Geometry check sheet. Reference: the model listing, model coordinates, mm. A direction names the side the tool comes from. Coordinates: 2 decimals unless noted, no trailing zeros. Write each loop counter-clockwise with the first axis right and the second up, starting at its lowest first coordinate (ties: lowest second). Pieces come first, ordered by that corner, then holes. Notation, with made-up numbers: M 76,-19 L 103,-19 A24 ccw 103,2 Z; hole C -36.5,61 d8. An arc over 180 degrees is marked long. Write each question's results on one line, items separated by ' | '.
```python
from build123d import *


with BuildPart() as part:
    # Sketch1 → Revolve1 (revolve)
    with BuildSketch(Plane.XY):
        with BuildLine():
            Line((1, 16.75), (0, 15.75))
            Line((0, 15.75), (0, 5.1))
            Line((0, 5.1), (15, 5.1))
            Line((15, 5.1), (15, 13.249667434))
            ThreePointArc((15, 13.249667434), (15.22452816, 13.805394131), (15.772080403, 14.049180096))
            Line((15.772080403, 14.049180096), (43, 15))
            Line((43, 15), (43, 19.5))
            ThreePointArc((43, 19.5), (42.121320344, 21.621320344), (40, 22.5))
            Line((40, 22.5), (9.28444402, 22.5))
            Line((9.28444402, 22.5), (5, 19.5))
            Line((5, 19.5), (5, 17.75))
            Line((5, 17.75), (3, 17.75))
            Line((3, 17.75), (3, 16.75))
            Line((3, 16.75), (1, 16.75))
        make_face()
    revolve(axis=Axis((0, 0, 0), (1, 0, 0)))


solid = part.part
```
Q1. Sectioned sample at A-A on y = 0. Record the cut outline in (x, z).
Geometry check:
outline: M 0,-15.75 L 1,-16.75 L 3,-16.75 L 3,-17.75 L 5,-17.75 L 5,-19.5 L 9.28,-22.5 L 40,-22.5 A3 ccw 43,-19.5 L 43,-15 L 15.77,-14.05 A0.8 cw 15,-13.25 L 15,-5.1 L 0,-5.1 Z; M 0,5.1 L 15,5.1 L 15,13.25 A0.8 cw 15.77,14.05 L 43,15 L 43,19.5 A3 ccw 40,22.5 L 9.28,22.5 L 5,19.5 L 5,17.75 L 3,17.75 L 3,16.75 L 1,16.75 L 0,15.75 Z
Q2. Scan lines: probe 1 along Z at (x, y) = (10, 0); probe 2 along Z at (x, y) = (7, 0); probe 3 along X at (y, z) = (-2.5, -5.5). Record each from-to range of solid material in increasing order.
Geometry check:
probe 1: z = -22.5 to -5.1, 5.1 to 22.5 | probe 2: z = -20.9 to -5.1, 5.1 to 20.9 | probe 3: x = 0 to 15
Q3. Sectioned sample at D-D on x = 25. Record the cut outline in (y, z), and give its area (3 significant figures).
Geometry check:
outline: C 0,0 d45; hole C 0,0 d28.74 | area: 942 mm2
Q4. Mould release check, pull along Z, two halves, no side actions. Record for faces 1 (the cylindrical face through (1.99, -3.63, -16.35)), 2 (the flat face through (15, 0, -6)), 3 (the flat face through (43, -10, -11.5)), 4 (the conical face through (29.577, -11.531, -8.842)): pulls with the +Z half, pulls with the -Z half, needs draft (parallel to the pull), parting line crosses it, or undercut.
Geometry check:
face 1: parting line crosses it | face 2: undercut | face 3: needs draft | face 4: undercut
Q5. Access from +Z, -Z, +X, -X, +Y, -Y to the whole of each face (thin tool, end or side, straight path). Record for faces 5 (the cylindrical face through (24.427, 10.382, -19.961)), 6 (the flat face through (5, 9, -16)).
Geometry check:
face 5: +X, -X | face 6: -X
Q6. Depth check by flat-ended pin: P1, Ø3, axis at x = 28.5, z = 3, coming from the -Y side; P2, Ø1, axis at y = -5.5, z = 8, coming from the +X side; P3, Ø1.5, axis at x = 6.5, z = -5.5, coming from the +Y side; P4, Ø6, axis at y = 0, z = 0, coming from the +X side. Enter the tip coordinate at first touch or a pass-through.
Geometry check:
P1: stops at y = -22.45 | P2: stops at x = 15 | P3: stops at y = 20.38 | P4: passes through
Q7. Sectioned sample at C-C on x = 19. Record the cut outline in (y, z), and give its area (3 significant figures).
Geometry check:
outline: C 0,0 d45; hole C 0,0 d28.32 | area: 960 mm2
